Autodesk Inventor part; units mm, degrees
ref_plane "Work Plane2" through (3.35, 0, 0) normal (0, 0, -1) x (1, 0, 0)
ref_plane "YZ Plane" through (0, 0, 0) normal (1, 0, 0) x (0, 1, 0)
ref_plane "XZ Plane" through (0, 0, 0) normal (0, 1, 0) x (-1, 0, 0)
sketch "Sketch1" plane through (0, 0, 0) normal (0, 0, 1) x (1, 0, 0)
  line L0 (1.7796, 0) -> (7.9375, 0)
  line L1 (7.9375, 0) -> (7.9375, 1.4224)
  line L2 (7.9375, 1.4224) -> (3.2893, 1.4224)
  line L3 (3.2893, 1.4224) -> (2.6543, 1.4224)
  line L4 (2.6543, 1.4224) -> (1.7018, 1.4224)
  line L5 (0, 2.4765) -> (0, 1.9939)
  line L6 (0, 1.9939) -> (0.979, 1.5058)
  line L7 (0.979, 1.5058) -> (1.7796, 0)
  line L8 (-1.5875, 0) -> (9.525, 0)
  line L9 (0, -0.4953) -> (0, 2.9718)
  line L10 (0, 2.4765) -> (0.4892, 2.4765)
  line L11 (0.4892, 2.4765) -> (1.7018, 1.4224)
  line L12 (3.2893, 1.4224) -> (1.7018, 1.4224) construction
  dimension "d1" = 4.6482
  dimension "d2" = 2.8448
  dimension "d3" = 2.8448
  dimension "d4" = 3.9878
  dimension "d5" = 26.5
  dimension "d6" = 62
  dimension "d7" = 1.7796
  dimension "d8" = 0.635
  dimension "d12" = 4.953
  dimension "d13" = 41
  dimension "d15" = 7.9375
  dimension "d24" = 1.7018
revolve "Body" add sketch "Sketch1" angle 360 about axis through (1.7796, 0, 0) along (1, 0, 0) contours L7 L6 L5 L10 L11 L4 L3 L2 L1 L0
sketch "Sketch2" plane through (0, 0, 0) normal (-1, 0, 0) x (0, 0, 1)
  line L0 (0, 1.9939) -> (0, 0) construction
  line L1 (0, 0) -> (1.9939, 0) construction
  arc A0 (0.5982, 0) -> (0, 0.5982) centre (0, 0) ccw construction
  arc A1 (0.6979, 0) -> (0, 0.6979) centre (0, 0) ccw construction
  arc A2 (1.952, 0.4064) -> (0.4064, 1.952) centre (0, 0) ccw
  line L2 (0, 0) -> (1.4099, 1.4099) construction
  line L3 (0.4064, 1.952) -> (0.3529, 0.6021)
  line L4 (1.952, 0.4064) -> (0.6021, 0.3529)
  arc A3 (0.4064, 1.952) -> (0, 1.9939) centre (0, 0) ccw
  arc A4 (1.9939, 0) -> (1.952, 0.4064) centre (0, 0) ccw
  line L5 (0, -3.4671) -> (0, 3.4671)
  line L6 (-3.4671, 0) -> (3.4671, 0)
  arc A5 (0.4064, -1.952) -> (1.952, -0.4064) centre (0, 0) ccw
  line L7 (0.4064, -1.952) -> (0.3529, -0.6021)
  line L8 (1.952, -0.4064) -> (0.6021, -0.3529)
  arc A6 (0, -1.9939) -> (0.4064, -1.952) centre (0, 0) ccw
  arc A7 (1.952, -0.4064) -> (1.9939, 0) centre (0, 0) ccw
  arc A8 (-0.4064, 1.952) -> (-1.952, 0.4064) centre (0, 0) ccw
  line L9 (-0.4064, 1.952) -> (-0.3529, 0.6021)
  line L10 (-1.952, 0.4064) -> (-0.6021, 0.3529)
  arc A9 (0, 1.9939) -> (-0.4064, 1.952) centre (0, 0) ccw
  arc A10 (-1.952, 0.4064) -> (-1.9939, 0) centre (0, 0) ccw
  arc A11 (-0.4064, -1.952) -> (0, -1.9939) centre (0, 0) ccw
  arc A12 (-1.952, -0.4064) -> (-0.4064, -1.952) centre (0, 0) ccw
  arc A13 (-1.9939, 0) -> (-1.952, -0.4064) centre (0, 0) ccw
  line L11 (-1.952, -0.4064) -> (-0.6021, -0.3529)
  line L12 (-0.4064, -1.952) -> (-0.3529, -0.6021)
  arc A14 (0.3529, 0.6021) -> (0.6021, 0.3529) centre (0.5926, 0.5926) ccw
  arc A15 (0.6021, -0.3529) -> (0.3529, -0.6021) centre (0.5926, -0.5926) ccw
  arc A16 (-0.6021, 0.3529) -> (-0.3529, 0.6021) centre (-0.5926, 0.5926) ccw
  arc A17 (-0.3529, -0.6021) -> (-0.6021, -0.3529) centre (-0.5926, -0.5926) ccw
  point P0 (1.4099, -1.4099)
  point P1 (-1.4099, 1.4099)
  point P2 (-1.4099, -1.4099)
  dimension "d17" = 1.1963
  dimension "d18" = 1.3957
  dimension "d19" = 3.9878
  dimension "d20" = 45
  dimension "d21" = 0.4064
extrude "Slot" add sketch "Sketch2" against normal up to next draft 5 contours L4 A14 L3 A2 | A5 L7 A15 L8 | L9 A16 L10 A8 | A12 L11 A17 L12
fillet "Fillet1" radius 0.1626 4 edges at (0, 1.9939, 0) (0, 0, -1.9939) (0, -1.9939, 0) (0, 0, 1.9939)
thread "Thread"
chamfer "Chamfer1" distance 0.4763 distance2 0.3175 1 edges at (7.9375, -1.4224, 0) measured on face at (7.9375, -0.4198, 0.2203)
ref_plane "Work Plane2" through (3.35, 0, 0) normal (0, 0, -1) x (1, 0, 0)
equation "\"d1\" = GEL"
equation "\"d2\" = GD"
equation "\"d3\" = BDM"
equation "\"d4\" = SDM"
equation "\"d7\" = INTI"
equation "\"d8\" = GAL"
equation "\"d12\" = KOD"
equation "\"d13\" = 0.5 * SEWI"
equation "\"d15\" = NLG"
equation "\"d24\" = KOH"
equation "\"d17\" = 0.3 * SDM"
equation "\"d18\" = 0.35 * SDM"
equation "\"d19\" = SDM"
equation "\"d21\" = 0.5 * SBR"
equation "\"d23\" = 0.2 * SBR"
equation "\"d10\" = GEL"
equation "\"d25\" = -0.5 * SPD + 0.5 * GD"
equation "\"d26\" = 0.5 * GAL"
equation "\"NLG\" = 7.9375"
equation "\"GEL\" = 4.6482"
equation "\"GAL\" = 0.635"
equation "\"SPD\" = 1.8923"
equation "\"KOD\" = 4.953"
equation "\"KOH\" = 1.7018"
equation "\"SBR\" = 0.8128"
equation "\"SDM\" = 3.9878"
equation "\"GD\" = NND"
equation "\"BDM\" = NND"
equation "\"SEWI\" = 82deg"
equation "\"d9\" = SDM"
equation "\"GUL\" = 0.75 * GAL"
equation "\"TOA\" = 30deg"
equation "\"THREADDIA\" = 2.8448"
equation "\"NND\" = 2.8448"
equation "\"INTI1\" = 2.2352"
equation "\"GD1\" = SPD"
properties part number "ANSI B18.6.3 - 4-40 x 5/16, CRFCHMSTII(3)" material "Steel, Mild"
Verification items for the finished model (mm, model axes). A direction names the side the tool comes from. Give positions to 0.01 mm unless a question says otherwise; leave off trailing zeros. Order: outer loops, then holes, each group sorted by start corner. A loop starts at its lowest first (then second) coordinate and runs counter-clockwise, first axis right, second up. Notation, with made-up numbers: (2, 39.5) -> (25, 39.5) arc R30 ccw to (25, 67.5) -> close; hole circle Ø9 at (73, -18.5). An arc over 180 degrees is marked (long way). Use a Markdown table: item, result.
1) Material ranges on probe 1 along X at (y, z) = (-1.75, -1.6); probe 2 along Y at (x, z) = (3.25, 0.05); probe 3 along Y at (x, z) = (7, 0.45), recorded low to high.
Results:
| item | result |
|---|---|
| probe 1 | 0 to 0.61 |
| probe 2 | -1.42 to 1.42 |
| probe 3 | -1.35 to 1.35 |
2) Mould release check, pull along Z, two halves, no side actions. Record for faces 1 (the flat face through (7.938, 0, 0)), 2 (the cylindrical face through (0.248, -0.322, 2.455)), 3 (the flat face through (0.548, -1.179, 0.328)): pulls with the +Z half, pulls with the -Z half, needs draft (parallel to the pull), parting line crosses it, or undercut.
Results:
| item | result |
|---|---|
| face 1 | needs draft |
| face 2 | parting line crosses it |
| face 3 | undercut |
3) Tool access check on faces 4 (the flat face through (0.548, -0.328, 1.179)), 5 (the flat face through (0, 1, -1)), 6 (the cylindrical face through (4.62, -0.31, 1.39)). Record the directions out of +Z, -Z, +X, -X, +Y, -Y that give a thin tool (end or side, any length) a straight path to the whole face; none if there is none.
Results:
| item | result |
|---|---|
| face 4 | -X |
| face 5 | +Z, -Z, -X, +Y, -Y |
| face 6 | +X |
4) Depth check by flat-ended pin: pin 1 Ø1 at (x, z) = (2.5, 0) entering from -Y; pin 2 Ø1 at (x, y) = (6.5, -0.5) entering from -Z; pin 3 Ø1 at (x, z) = (1, -1.5) entering from -Y. Enter the tip coordinate at first touch or a pass-through.
Results:
| item | result |
|---|---|
| pin 1 | y = -1.42 |
| pin 2 | z = -1.42 |
| pin 3 | y = -2.06 |
5) Section check A-A, the plane x = 6.5. Record the boundary of the cut face in (y, z).
Results:
| item | result |
|---|---|
| outline | circle Ø2.84 at (0, 0) |
